Input: dimensioned drawing with shaded views. Units: mm. Origin: part minimum x, y, z. A direction names the side the tool comes from. Give positions to 0.01 mm unless a question says otherwise; leave off trailing zeros. Write each loop counter-clockwise with the first axis right and the second up, starting at its lowest first coordinate (ties: lowest second). Pieces come first, ordered by that corner, then holes. Notation, with made-up numbers: M 78.5,6.25 L 111.5,6.25 A28 ccw 111.5,45.25 Z; hole C 13.5,-36 d7. An arc over 180 degrees is marked long. Answer as a JSON object with one key per item and string values.
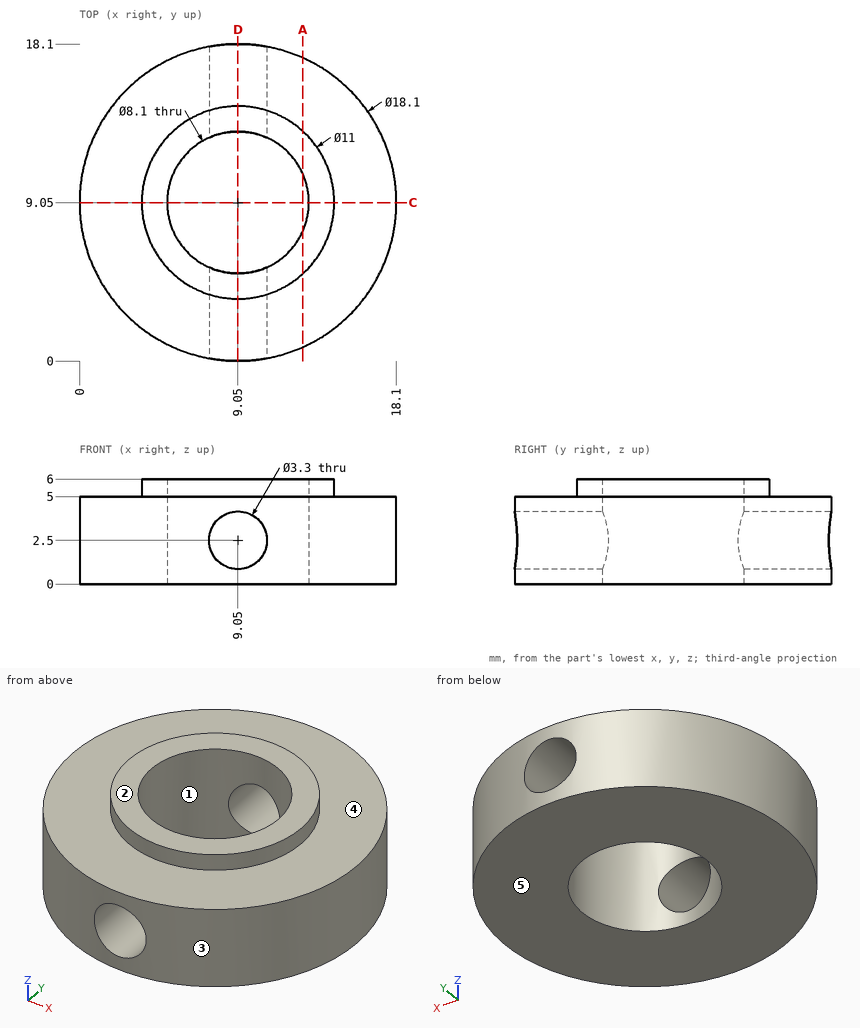
1) Cut plane D-D on x = 9.05. Return loops of the section in (y, z).
Geometry check:
{"outline": "M 0,0 L 5,0 L 5,0.85 L 0,0.85 Z; M 0,4.15 L 5,4.15 L 5,6 L 3.55,6 L 3.55,5 L 0,5 Z; M 13.1,0 L 18.1,0 L 18.1,0.85 L 13.1,0.85 Z; M 13.1,4.15 L 18.1,4.15 L 18.1,5 L 14.55,5 L 14.55,6 L 13.1,6 Z"}
2) Cut plane C-C on y = 9.05. Return loops of the section in (x, z).
Geometry check:
{"outline": "M 0,0 L 5,0 L 5,6 L 3.55,6 L 3.55,5 L 0,5 Z; M 13.1,0 L 18.1,0 L 18.1,5 L 14.55,5 L 14.55,6 L 13.1,6 Z"}
3) Line query: line 1 (Y direction, x = 9.05, z = 4.5); line 2 (X direction, y = 7, z = 4); line 3 (Z direction, x = 3.25, y = 9.5). Output: solid intervals per line, ascending. Write a range as from..to.
Geometry check:
{"line 1": "y = 0..5, 13.1..18.1", "line 2": "x = 0.24..5.56, 12.54..17.86", "line 3": "z = 0..5"}
4) Set-up query: the marked faces 4 and 5. Return all of +Z, -Z, +X, -X, +Y, -Y with unobstructed straight access to the full face (end or side cutting, diameter ignored); none if empty.
Geometry check:
{"face 4": "+Z", "face 5": "-Z, +X, -X, +Y, -Y"}
5) Cut plane A-A on x = 12.75. Return loops of the section in (y, z), and give its area (3 significant figures).
Geometry check:
{"outline": "M 0.79,0 L 7.4,0 L 7.4,6 L 4.98,6 L 4.98,5 L 0.79,5 Z; M 10.7,0 L 17.31,0 L 17.31,5 L 13.12,5 L 13.12,6 L 10.7,6 Z", "area": "71.0 mm2"}
6) Pull-direction query (X, two-part tool) for the marked faces 1, 2 and 3; classes: pulls with the +X half, pulls with the -X half, needs draft (parallel to the pull), parting line crosses it, or undercut.
Geometry check:
{"face 1": "undercut", "face 2": "needs draft", "face 3": "parting line crosses it"}
7) Contact query for flat-ended pins moving along their axis: P1, Ø3, axis at x = 9.05, z = 2.5, coming from the -Y side; P2, Ø1.5, axis at y = 14, z = 4, coming from the +X side; P3, Ø5.5, axis at x = 8, y = 6, coming from the +Z side. Output: stop coordinate, or through.
Geometry check:
{"P1": "passes through", "P2": "stops at x = 17.07", "P3": "stops at z = 6"}
